from build123d import *

# Parameters (mm, degrees)
F0_R     = 2.175
F1_DEPTH = 8.3
F2_R     = 2.175
F3_DEPTH = 4


with BuildPart() as f1:
    # F0 (on Top) → F1 (new body)
    with BuildSketch(Plane.XY):
        Circle(F0_R)
    extrude(amount=F1_DEPTH)

    # F2 (on face) → F3 (join)
    with BuildSketch(Plane.XY.offset(8.3)):
        Polygon((5.26072, -6.895255), (8.595572, -1.15579), (6.895255, 5.26072), (1.15579, 8.595572), (-5.26072, 6.895255), (-8.595572, 1.15579), (-6.895255, -5.26072), (-1.15579, -8.595572), align=None)
        Circle(F2_R, mode=Mode.SUBTRACT)
        Circle(F2_R)
    extrude(amount=F3_DEPTH)


solid = f1.part
Here's how the part is built. I have some questions about the finished solid (model axes, mm). A direction names the side the tool comes from. Coordinates: 2 decimals unless noted, no trailing zeros. Loops run counter-clockwise (first coordinate to the right, second up) from the corner with the lowest first, then second, coordinate; pieces in that order, holes last.
1. I need wall thicknesses on L1, parallel to Z at x = 1.25, y = 3.5; L2, parallel to X at y = 1, z = 1.75; L3, parallel to Y at x = -1.75, z = 6. Which ranges of each line are inside material? Lowest first, please.
2. Imagine slicing it at D-D, the plane z = 3.75. Please give me the cut outline in (x, y) (3 decimals).
3. Imagine slicing it at A-A, the plane z = 9. Please give me the cut outline in (x, y).
4. Imagine slicing it at C-C, the plane y = -6.25. Please give me the cut outline in (x, z).
5. For faces 1 (the flat face through (-6.9, 4.07, 10.27)), 2 (the flat face through (2, -2, 8.3)), which set-ups out of +Z, -Z, +X, -X, +Y, -Y let a thin tool reach every point of the face, with its end or its side?
6. Imagine slicing it at B-B, the plane x = -1.75. Please give me the cut outline in (y, z).
7. For P1, Ø5, axis at y = 4, z = 10, coming from the +X side; P2, Ø3, axis at y = 3, z = 9.5, coming from the -X side, each with a flat end and sliding along its axis, tell me the tip position at first contact or that it passes through.
Taken from the geometry:
1. L1: z = 8.3 to 12.3
1. L2: x = -1.93 to 1.93
1. L3: y = -1.29 to 1.29
2. outline: circle Ø4.35 at (0, 0)
3. outline: (-8.6, 1.16) - (-6.9, -5.26) - (-1.16, -8.6) - (5.26, -6.9) - (8.6, -1.16) - (6.9, 5.26) - (1.16, 8.6) - (-5.26, 6.9) - close
4. outline: (-5.19, 8.3) - (5.64, 8.3) - (5.64, 12.3) - (-5.19, 12.3) - close
5. face 1: +Z, -Z, -X, +Y
5. face 2: -Z
6. outline: (-8.25, 8.3) - (-1.29, 8.3) - (-1.29, 0) - (1.29, 0) - (1.29, 8.3) - (7.83, 8.3) - (7.83, 12.3) - (-8.25, 12.3) - close
7. P1: stops at x = 7.89
7. P2: stops at x = -8.4
